Autodesk Inventor part; units mm, degrees
ref_plane "YZ Plane" through (0, 0, 0) normal (1, 0, 0) x (0, 1, 0)
ref_plane "XZ Plane" through (0, 0, 0) normal (0, 1, 0) x (-1, 0, 0)
ref_plane "XY Plane" through (0, 0, 0) normal (0, 0, 1) x (1, 0, 0)
sketch "Sketch1" plane through (0, 0, 0) normal (0, 1, 0) x (-1, 0, 0)
  line L0 (27.25, 27.25) -> (-27.25, 27.25)
  line L1 (-27.25, 27.25) -> (-27.25, -27.25)
  line L2 (-27.25, -27.25) -> (27.25, -27.25)
  line L3 (27.25, -27.25) -> (27.25, 27.25)
  line L4 (27.25, 27.25) -> (-27.25, -27.25) construction
  line L5 (-27.25, 27.25) -> (27.25, -27.25) construction
  line L6 (21, 21) -> (-21, 21)
  line L7 (-21, 21) -> (-21, -21)
  line L8 (-21, -21) -> (21, -21)
  line L9 (21, -21) -> (21, 21)
  line L10 (21, 21) -> (-21, -21) construction
  line L11 (-21, 21) -> (21, -21) construction
  point P0 (0, 0)
  dimension "d0" = 54.5
  dimension "d1" = 54.5
  dimension "d2" = 42
  dimension "d3" = 42
extrude "Extrusion1" add sketch "Sketch1" along normal blind 6 contours L3 L2 L1 L0 | L9 L8 L7 L6
sketch "Sketch2" plane through (0, 6, 0) normal (0, 1, 0) x (1, 0, 0)
  circle A0 centre (0, 0) radius 25
  dimension "d7" = 50
extrude "Extrusion2" add sketch "Sketch2" along normal blind 2.5
sketch "Sketch3" plane through (0, 0, 0) normal (0, -1, 0) x (1, 0, 0)
  circle A0 centre (0, 0) radius 26
  dimension "d10" = 52
extrude "Extrusion3" add sketch "Sketch3" along normal blind 126
fillet "Fillet1" radius 2.5 1 edges at (-26, -126, 0)
fillet "Fillet2" radius 2 4 edges at (27.25, 3, -27.25) (-27.25, 3, -27.25) (-27.25, 3, 27.25) (27.25, 3, 27.25)
hole "Hole1" at (21, 0, -21) at (21, 0, 21) at (-21, 0, -21) at (-21, 0, 21) direction (0, 1, 0) diameter 4.4 end through all
sketch "Sketch4" plane through (0, 8.5, 0) normal (0, 1, 0) x (1, 0, 0)
  circle A0 centre (0, 0) radius 4
  dimension "d22" = 8
extrude "Extrusion4" add sketch "Sketch4" along normal blind 25
equation "\"d1\" = d0"
equation "\"d3\" = d2"
properties part number "Nanotec-DH038-Servo"
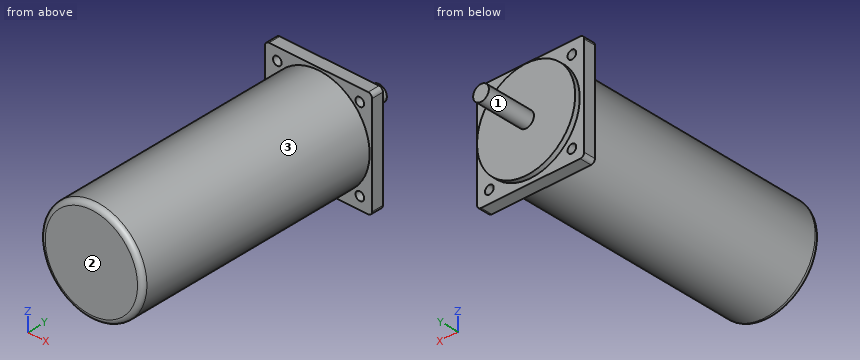
Can you work these out from the model? Positions are in its coordinate system, mm. Face numbers are marked on the shaded views. A direction names the side the tool comes from. Coordinates: 2 decimals unless noted, no trailing zeros. Write each loop counter-clockwise with the first axis right and the second up, starting at its lowest first coordinate (ties: lowest second). Pieces come first, ordered by that corner, then holes. Notation, with made-up numbers: (8, 68) - (31, 68) arc R36 cw to (31, 107) - close; hole circle Ø10 at (64.5, -3.5). An arc over 180 degrees is marked (long way). Return JSON: item names as keys, results as strings. Group by question number.
Item 1: I'm going to push flat-ended pins straight in: pin 1 Ø7 at (x, z) = (-21, -21) entering from -Y; pin 2 Ø4 at (x, y) = (3.5, -76.5) entering from +Z; pin 3 Ø16.5 at (x, z) = (-12, 7.5) entering from +Y; pin 4 Ø2.5 at (x, z) = (-21, 21) entering from -Y. Where does each tip first touch, or does it pass through?
Item 2: If we section it at A-A (x = 0): Write out the boundary of the cut face in (y, z).
Item 3: Please list where these lines run through material, in increasing order: probe 1 along Z at (x, y) = (-21, 2.8); probe 2 along Y at (x, z) = (-21.5, -10).
Item 4: If we section it at C-C (z = -21): Count the separate pieces of the cut face and the enclosed holes in it, then the cut area to 3 significant figures.
Item 5: Which directions (+Z, -Z, +X, -X, +Y, -Y) give clear straight access to the entire face, cutting with the end or side of a thin tool? Please do the marked faces 1, 2 and 3.
Item 6: If we section it at B-B (y = 14): Write out the boundary of the cut face in (x, z), then the cut area to 3 significant figures.
Return value:
{
 "1": {"pin 1": "stops at y = 0", "pin 2": "stops at z = 25.96", "pin 3": "stops at y = 8.5", "pin 4": "passes through"},
 "2": {"outline": "(-126, -23.5) arc R2.5 ccw to (-123.5, -26) - (0, -26) - (0, -27.25) - (6, -27.25) - (6, -25) - (8.5, -25) - (8.5, -4) - (33.5, -4) - (33.5, 4) - (8.5, 4) - (8.5, 25) - (6, 25) - (6, 27.25) - (0, 27.25) - (0, 26) - (-123.5, 26) arc R2.5 ccw to (-126, 23.5) - close"},
 "3": {"probe 1": "z = -27.25 to -23.2, -18.8 to 18.8, 23.2 to 27.25", "probe 2": "y = -125.99 to 8.5"},
 "4": {"separate pieces": "3", "enclosed holes": "0", "area": "4,200 mm^2"},
 "5": {"face 1": "+Y", "face 2": "+Z, -Z, +X, -X, -Y", "face 3": "-Y"},
 "6": {"outline": "circle Ø8 at (0, 0)", "area": "50.3 mm^2"}
}
